Work out the finished part from the listing and answer in its coordinate system (mm). Face numbers are marked on the shaded views. A direction names the side the tool comes from. Coordinates: 2 decimals unless noted, no trailing zeros. Loops run counter-clockwise (first coordinate to the right, second up) from the corner with the lowest first, then second, coordinate; pieces in that order, holes last. Notation, with made-up numbers: (-3.5, -10) -> (35.5, -10) arc R23 ccw to (35.5, -1) -> close; hole circle Ø2 at (38.5, 24). An arc over 180 degrees is marked (long way). Use a Markdown table: item, result.
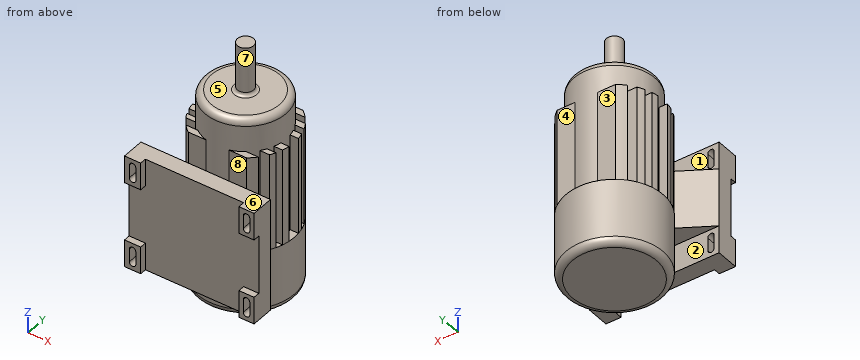
from build123d import *
from build123d.topology import SkipClean

# Parameters (mm, degrees)
SKETCH1_R            = 150
BOSS_EXTRUDE1_DEPTH  = 200
BOSS_EXTRUDE11_DEPTH = 300
BOSS_EXTRUDE14_START = -300
SKETCH12_R           = 125
BOSS_EXTRUDE14_DEPTH = 400
SKETCH13_W           = 46.677917496
SKETCH13_H           = 84.453402707
SKETCH13_H_2         = 84.453402706
SKETCH13_W_2         = 50
BOSS_EXTRUDE15_DEPTH = 50
SKETCH13_3_W         = 46.677917496
SKETCH13_3_H         = 84.453402706
SKETCH13_3_H_2       = 84.453402707
SKETCH13_3_W_2       = 50
BOSS_EXTRUDE16_DEPTH = 20
BOSS_EXTRUDE17_DEPTH = 90
SKETCH16_R           = 25
BOSS_EXTRUDE18_DEPTH = 150
FILLET2_R            = 10
FILLET3_R            = 20
SCALE4_SCALE         = 0.22917


with BuildPart() as part:
    # Sketch1 → Boss-Extrude1 (new body)
    with BuildSketch(Plane.XY):
        Circle(SKETCH1_R)
    extrude(amount=BOSS_EXTRUDE1_DEPTH)

    # Sketch7 → Boss-Extrude11 (add)
    with SkipClean():  # the faces are left unmerged after this step: merging them gives an invalid solid
        with BuildSketch(Plane.XY.offset(200)):
            with BuildLine():
                Line((-90, 120), (90, 120))
                ThreePointArc((90, 120), (101.396020382, 110.538893837), (111.803398875, 100))
                Line((111.803398875, 100), (-111.803398875, 100))
                ThreePointArc((-111.803398875, 100), (-101.396020382, 110.538893837), (-90, 120))
            make_face()
            with BuildLine():
                Line((-126.885775404, 80), (126.885775404, 80))
                ThreePointArc((126.885775404, 80), (132.559251115, 70.200035213), (137.477270849, 60))
                Line((137.477270849, 60), (-137.477270849, 60))
                ThreePointArc((-137.477270849, 60), (-132.559251115, 70.200035213), (-126.885775404, 80))
            make_face()
            with BuildLine():
                Line((144.16342013, -41.435592144), (-144.16342013, -41.435592144))
                ThreePointArc((-144.16342013, -41.435592144), (-146.803816882, -30.799989431), (-148.660687473, -20))
                Line((-148.660687473, -20), (148.660687473, -20))
                ThreePointArc((148.660687473, -20), (146.803816882, -30.799989431), (144.16342013, -41.435592144))
            make_face()
            with BuildLine():
                Line((111.803398875, -100), (-111.803398875, -100))
                ThreePointArc((-111.803398875, -100), (-101.396020382, -110.538893837), (-90, -120))
                Line((-90, -120), (90, -120))
                ThreePointArc((90, -120), (101.396020382, -110.538893837), (111.803398875, -100))
            make_face()
            with BuildLine():
                Line((144.568322948, 40), (-144.568322948, 40))
                ThreePointArc((-144.568322948, 40), (-146.955139883, 30.069700063), (-148.660687473, 20))
                Line((-148.660687473, 20), (148.660687473, 20))
                ThreePointArc((148.660687473, 20), (146.955139883, 30.069700063), (144.568322948, 40))
            make_face()
            with BuildLine():
                Line((137.477270849, -60), (-137.477270849, -60))
                ThreePointArc((-137.477270849, -60), (-133.599215205, -68.20007109), (-129.232599216, -76.150740639))
                Line((-129.232599216, -76.150740639), (129.232599216, -76.150740639))
                ThreePointArc((129.232599216, -76.150740639), (133.599215205, -68.20007109), (137.477270849, -60))
            make_face()
        extrude(amount=BOSS_EXTRUDE11_DEPTH)



with BuildPart() as body_2:
    # Sketch12 → Boss-Extrude14 (new body)
    with BuildSketch(Plane.XY.offset(500).offset(BOSS_EXTRUDE14_START)):
        Circle(SKETCH12_R)
    extrude(amount=BOSS_EXTRUDE14_DEPTH)


with BuildPart() as body_3:
    # Sketch13 → Boss-Extrude15 (new body)
    # profile 1 of 5: a face of its own
    with BuildSketch(Plane(origin=(0, -220, 0), x_dir=(-1, 0, 0), z_dir=(0, -1, 0))):
        Polygon((150, -99.735715433), (-153.322082504, -99.735715433), (-153.322082504, -184.18911814), (-200, -184.18911814), (-200, -365.282312727), (-153.322082504, -365.282312727), (-153.322082504, -449.735715433), (150, -449.735715433), (150, -365.282312727), (200, -365.282312727), (200, -184.18911814), (150, -184.18911814), align=None)
    # profile 2 of 5: a face of its own
    with BuildSketch(Plane(origin=(0, -220, 0), x_dir=(-1, 0, 0), z_dir=(0, -1, 0))):
        with Locations((-176.661041252, -141.962416787)):
            Rectangle(SKETCH13_W, SKETCH13_H)
        with BuildLine():
            ThreePointArc((-186.661041252, -121.962416787), (-176.661041252, -111.962416787), (-166.661041252, -121.962416787))
            Line((-166.661041252, -121.962416787), (-166.661041252, -161.962416787))
            ThreePointArc((-166.661041252, -161.962416787), (-176.661041252, -171.962416787), (-186.661041252, -161.962416787))
            Line((-186.661041252, -161.962416787), (-186.661041252, -121.962416787))
        make_face(mode=Mode.SUBTRACT)
    # profile 3 of 5: a face of its own
    with BuildSketch(Plane(origin=(0, -220, 0), x_dir=(-1, 0, 0), z_dir=(0, -1, 0))):
        with Locations((-176.661041252, -407.50901408)):
            Rectangle(SKETCH13_W, SKETCH13_H_2)
        with BuildLine():
            Line((-166.661041252, -387.50901408), (-166.661041252, -427.50901408))
            ThreePointArc((-166.661041252, -427.50901408), (-176.661041252, -437.50901408), (-186.661041252, -427.50901408))
            Line((-186.661041252, -427.50901408), (-186.661041252, -387.50901408))
            ThreePointArc((-186.661041252, -387.50901408), (-176.661041252, -377.50901408), (-166.661041252, -387.50901408))
        make_face(mode=Mode.SUBTRACT)
    # profile 4 of 5: a face of its own
    with BuildSketch(Plane(origin=(0, -220, 0), x_dir=(-1, 0, 0), z_dir=(0, -1, 0))):
        with Locations((175, -407.50901408)):
            Rectangle(SKETCH13_W_2, SKETCH13_H_2)
        with BuildLine():
            Line((185, -387.50901408), (185, -427.50901408))
            ThreePointArc((185, -427.50901408), (175, -437.50901408), (165, -427.50901408))
            Line((165, -427.50901408), (165, -387.50901408))
            ThreePointArc((165, -387.50901408), (175, -377.50901408), (185, -387.50901408))
        make_face(mode=Mode.SUBTRACT)
    # profile 5 of 5: a face of its own
    with BuildSketch(Plane(origin=(0, -220, 0), x_dir=(-1, 0, 0), z_dir=(0, -1, 0))):
        with Locations((175, -141.962416787)):
            Rectangle(SKETCH13_W_2, SKETCH13_H)
        with BuildLine():
            ThreePointArc((165, -121.962416787), (175, -111.962416787), (185, -121.962416787))
            Line((185, -121.962416787), (185, -161.962416787))
            ThreePointArc((185, -161.962416787), (175, -171.962416787), (165, -161.962416787))
            Line((165, -161.962416787), (165, -121.962416787))
        make_face(mode=Mode.SUBTRACT)
    extrude(amount=-BOSS_EXTRUDE15_DEPTH)

    # Sketch13<3> → Boss-Extrude16 (add)
    # profile 1 of 4: a face of its own
    with BuildSketch(Plane(origin=(0, -220, 0), x_dir=(-1, 0, 0), z_dir=(0, -1, 0))):
        with Locations((-176.661041252, -407.50901408)):
            Rectangle(SKETCH13_3_W, SKETCH13_3_H)
        with BuildLine():
            Line((-166.661041252, -387.50901408), (-166.661041252, -427.50901408))
            ThreePointArc((-166.661041252, -427.50901408), (-176.661041252, -437.50901408), (-186.661041252, -427.50901408))
            Line((-186.661041252, -427.50901408), (-186.661041252, -387.50901408))
            ThreePointArc((-186.661041252, -387.50901408), (-176.661041252, -377.50901408), (-166.661041252, -387.50901408))
        make_face(mode=Mode.SUBTRACT)
    # profile 2 of 4: a face of its own
    with BuildSketch(Plane(origin=(0, -220, 0), x_dir=(-1, 0, 0), z_dir=(0, -1, 0))):
        with Locations((-176.661041252, -141.962416787)):
            Rectangle(SKETCH13_3_W, SKETCH13_3_H_2)
        with BuildLine():
            ThreePointArc((-186.661041252, -121.962416787), (-176.661041252, -111.962416787), (-166.661041252, -121.962416787))
            Line((-166.661041252, -121.962416787), (-166.661041252, -161.962416787))
            ThreePointArc((-166.661041252, -161.962416787), (-176.661041252, -171.962416787), (-186.661041252, -161.962416787))
            Line((-186.661041252, -161.962416787), (-186.661041252, -121.962416787))
        make_face(mode=Mode.SUBTRACT)
    # profile 3 of 4: a face of its own
    with BuildSketch(Plane(origin=(0, -220, 0), x_dir=(-1, 0, 0), z_dir=(0, -1, 0))):
        with Locations((175, -407.50901408)):
            Rectangle(SKETCH13_3_W_2, SKETCH13_3_H)
        with BuildLine():
            Line((185, -387.50901408), (185, -427.50901408))
            ThreePointArc((185, -427.50901408), (175, -437.50901408), (165, -427.50901408))
            Line((165, -427.50901408), (165, -387.50901408))
            ThreePointArc((165, -387.50901408), (175, -377.50901408), (185, -387.50901408))
        make_face(mode=Mode.SUBTRACT)
    # profile 4 of 4: a face of its own
    with BuildSketch(Plane(origin=(0, -220, 0), x_dir=(-1, 0, 0), z_dir=(0, -1, 0))):
        with Locations((175, -141.962416787)):
            Rectangle(SKETCH13_3_W_2, SKETCH13_3_H_2)
        with BuildLine():
            ThreePointArc((165, -121.962416787), (175, -111.962416787), (185, -121.962416787))
            Line((185, -121.962416787), (185, -161.962416787))
            ThreePointArc((185, -161.962416787), (175, -171.962416787), (165, -161.962416787))
            Line((165, -161.962416787), (165, -121.962416787))
        make_face(mode=Mode.SUBTRACT)
    extrude(amount=BOSS_EXTRUDE16_DEPTH)


with BuildPart() as part_1:
    with SkipClean():  # the faces are left unmerged after this step: merging them gives an invalid solid
        add(part.part)

        add(body_2.part)  # Boss-Extrude17 merges body 2

        add(body_3.part)  # Boss-Extrude17 merges body 3
        # Sketch14 → Boss-Extrude17 (add, symmetric)
        with BuildSketch(Plane.XY.offset(274.735715433)):
            Polygon((-200, -170), (200, -170), (100, -110), (-100, -110), align=None)
        extrude(amount=BOSS_EXTRUDE17_DEPTH, both=True)

    # Sketch16 → Boss-Extrude18 (add)
    with BuildSketch(Plane.XY.offset(600)):
        Circle(SKETCH16_R)
    extrude(amount=BOSS_EXTRUDE18_DEPTH)

    # Fillet2
    fillet2_edges = [part_1.edges().sort_by_distance(p)[0] for p in [
        (-25, 0, 600),
    ]]
    fillet(fillet2_edges, radius=FILLET2_R)

    # Fillet3
    fillet3_edges = [part_1.edges().sort_by_distance(p)[0] for p in [
        (-125, 0, 600),
        (-150, 0, 0),
    ]]
    fillet(fillet3_edges, radius=FILLET3_R)


with BuildPart() as part_2:
    # Scale4: scaled about (-0.042581341, -38.738063296, 280.973660068)
    add(part_1.part.scale(SCALE4_SCALE).moved(Location((-0.032822975, -29.86046133, 216.58292639))))


solid = part_2.part
Q1. Determine the mould class of the marked faces 6, 7 and 8 for opening direction Y: pulls with the +Y half, pulls with the -Y half, needs draft (parallel to the pull), parting line crosses it, or undercut.
Solved:
| item | result |
|---|---|
| face 6 | needs draft |
| face 7 | parting line crosses it |
| face 8 | undercut |
Q2. Section A-A on z = 335.5 is taken. Determine the outline of the cut face in (x, y), and give its area (3 significant figures).
Solved:
| item | result |
|---|---|
| outline | circle Ø57.29 at (-0.03, -29.86) |
| area | 2,580 mm² |
Q3. For the marked faces 1, 2, 3, 4 and 5, determine the directions among +Z, -Z, +X, -X, +Y, -Y from which every point of the face is accessible in a straight line to the end or side of a thin tool.
Solved:
| item | result |
|---|---|
| face 1 | +Z, +X, -X |
| face 2 | -Z, +X, -X |
| face 3 | +Z, -X, +Y |
| face 4 | +Z, +X, +Y |
| face 5 | +Z |
Q4. Consider line 1 (Y direction, x = -25.5, z = 317.5); line 2 (Y direction, x = 24, z = 283); line 3 (Z direction, x = -37.5, y = -64.5). Determine where each line is inside the solid, lowest interval first. Write a range as [from, to].
Solved:
| item | result |
|---|---|
| line 1 | [-80.28, -68.82], [-52.95, -52.78], [-47.31, -43.61], [-42.98, -16.74], [-16.11, -11.53], [-6.94, -6.77] |
| line 2 | [-80.28, -55.74], [-54.44, -52.78], [-47.31, -11.53], [-6.94, -5.28] |
| line 3 | [258.92, 300.17] |
Q5. Given pin 1 Ø1.4 at (x, y) = (29, -24) entering from +Z; pin 2 Ø2.5 at (x, y) = (21, -8.5) entering from +Z; pin 3 Ø6 at (x, y) = (29, -46) entering from -Z, each flat-ended and moving along its own axis, determine where each tip first touches the part or whether it passes through.
Solved:
| item | result |
|---|---|
| pin 1 | z = 331.17 |
| pin 2 | z = 262.42 |
| pin 3 | z = 216.6 |
